```python
from build123d import *

# Parameters (mm, degrees)
SKETCH2_W                       = 30
SKETCH2_H                       = 15
BOSS_EXTRUDE1_DEPTH             = 1
SKETCH4_W                       = 14.98037952
SKETCH4_H                       = 260
BOSS_EXTRUDE2_DEPTH             = 1
SKETCH6_W                       = 14.958437981
SKETCH6_H                       = 1
BOSS_EXTRUDE3_DEPTH             = 12
BOSS_EXTRUDE3_DIRECTION_2_REACH = 291.054


with BuildPart() as part:
    # Sketch2 → Boss-Extrude1 (new body)
    with BuildSketch(Plane(origin=(0, 0, 0), x_dir=(1, 0, 0), z_dir=(0, 1, 0))):
        with Locations((15, 7.5)):
            Rectangle(SKETCH2_W, SKETCH2_H)
    extrude(amount=BOSS_EXTRUDE1_DEPTH)

    # Sketch4 → Boss-Extrude2 (add)
    with BuildSketch(Plane(origin=(3.509333353, -9.641814145, 0), x_dir=(0, 0, -1), z_dir=(0.34202014332566616, -0.9396926207859094, 0))):
        with Locations((7.49018976, 158.190778624)):
            Rectangle(SKETCH4_W, SKETCH4_H)
    extrude(amount=-BOSS_EXTRUDE2_DEPTH)

    # Sketch6 → Boss-Extrude3 (add)
    with BuildSketch(Plane(origin=(274.320081404, 0, 0), x_dir=(0, 0, 1), z_dir=(1, 0, 0))):
        with Locations((-7.479218991, -89.425237265)):
            Rectangle(SKETCH6_W, SKETCH6_H)
    extrude(amount=BOSS_EXTRUDE3_DEPTH)

    # Boss-Extrude3 direction 2: up to this face of the body (flat: up to its plane)
    boss_extrude3_direction_2_end = Plane(part.part.faces().sort_by_distance((274.149071333, 89.395083575, -7.49018976))[0])
    # Sketch6 → Boss-Extrude3 direction 2 (add, up to the picked face)
    with BuildSketch(Plane(origin=(274.320081404, 0, 0), x_dir=(0, 0, 1), z_dir=(1, 0, 0)), mode=Mode.PRIVATE) as boss_extrude3_direction_2_sk1:
        with Locations((-7.479218991, -89.425237265)):
            Rectangle(SKETCH6_W, SKETCH6_H)
    boss_extrude3_direction_2_tool1 = split(extrude(boss_extrude3_direction_2_sk1.sketch, amount=-BOSS_EXTRUDE3_DIRECTION_2_REACH, mode=Mode.PRIVATE), bisect_by=boss_extrude3_direction_2_end, keep=Keep.BOTH, mode=Mode.PRIVATE)
    add(boss_extrude3_direction_2_tool1.solids().sort_by(Axis((274.320081, 89.425237, -7.479219), (-1, 0, 0)))[0])


solid = part.part
```
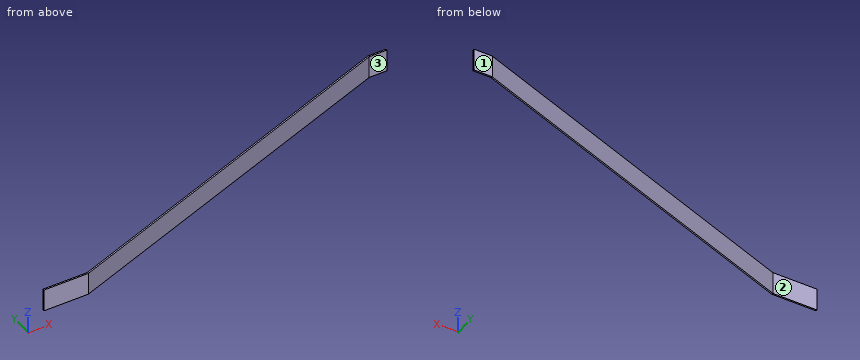
The model under review builds one solid part; all positions refer to its coordinate system, in mm. Face numbers are marked on the shaded views. A direction names the side the tool comes from. Round coordinates to 2 decimals unless told otherwise and drop trailing zeros. Order: outer loops, then holes, each group sorted by start corner. A loop starts at its lowest first (then second) coordinate and runs counter-clockwise, first axis right, second up. Notation, with made-up numbers: M 73,16 L 90,16 A12 ccw 90,37 Z; hole C -7.75,58.25 d9. An arc over 180 degrees is marked long. Use a Markdown table: item, result.
1) Insertion check: pin 1 (2 mm diameter, centred on x = 81.5, z = -1.5, fed in from +Y); pin 2 (1.1 mm diameter, centred on x = 283, y = 89.5, fed in from -Z); pin 3 (3.5 mm diameter, centred on x = 281, z = -8, fed in from -Y). Each pin has a flat end and moves straight along its axis. Give the tip position at first contact, or say it passes through.
Report:
| item | result |
|---|---|
| pin 1 | y = 20.17 |
| pin 2 | z = -14.96 |
| pin 3 | y = 88.93 |
2) Consider section A-A (z = -5.5). Write out the cut boundary in (x, y), then the cut area to 3 significant figures.
Report:
| item | result |
|---|---|
| outline | M 0,0 L 30,0 L 274.32,88.93 L 286.32,88.93 L 286.32,89.93 L 273.96,89.93 L 273.98,89.86 L 29.82,1 L 0,1 Z |
| area | 302 mm^2 |
3) Tool access review of the marked faces 1, 2 and 3: name each direction out of +Z, -Z, +X, -X, +Y, -Y from which nothing blocks a thin tool from reaching the whole face with its end or side.
Report:
| item | result |
|---|---|
| face 1 | +Z, -Z, +X, -X, +Y |
| face 2 | +Z, -Z, -X, +Y |
| face 3 | +Z, -Z, +X, -Y |
4) Consider section C-C (x = 243). Write out the cut boundary in (y, z).
Report:
| item | result |
|---|---|
| outline | M 77.53,-14.98 L 78.59,-14.98 L 78.59,0 L 77.53,0 Z |
5) Consider section B-B (y = 83). Write out the cut boundary in (x, z), then the cut area to 3 significant figures.
Report:
| item | result |
|---|---|
| outline | M 255.12,-14.98 L 258.04,-14.98 L 258.04,0 L 255.12,0 Z |
| area | 43.8 mm^2 |
6) Wall thickness on line 1 along Y through (x, z) = (221, -11.75); line 2 along Y through (x, z) = (54.5, -13.5): over which ranges is each line inside the solid? List them lowest first. Write a range as [from, to].
Report:
| item | result |
|---|---|
| line 1 | [69.52, 70.58] |
| line 2 | [8.92, 9.98] |
